```python
from build123d import *

# Parameters (mm, degrees)
SKETCH027_R     = 1.25
PAD016_DEPTH    = 5.3
SKETCH028_R     = 3.535534
SKETCH028_R_2   = 3.716517
POCKET008_DEPTH = 1.3
SKETCH032_W     = 20
SKETCH032_H     = 3
PAD019_DEPTH    = 8


with BuildPart() as part:
    # Sketch027 (on Face1 of ReferencePad002001) → Pad016 (new body)
    with BuildSketch(Plane.XY.offset(3.5)):
        Polygon((10, 124.725), (-10, 124.725), (-10, 129.975), (-25, 129.975), (-25, 134.475), (-10, 134.475), (-10, 139.725), (-10, 146.675), (10, 146.675), (10, 139.725), (10, 134.475), (25, 134.475), (25, 129.975), (10, 129.975), align=None)
        with Locations((7.5, 137.225)):
            Circle(SKETCH027_R, mode=Mode.SUBTRACT)
        with Locations((7.5, 127.225)):
            Circle(SKETCH027_R, mode=Mode.SUBTRACT)
        with Locations((-7.5, 127.225)):
            Circle(SKETCH027_R, mode=Mode.SUBTRACT)
        with Locations((-7.5, 137.225)):
            Circle(SKETCH027_R, mode=Mode.SUBTRACT)
        with Locations((-20, 132.225)):
            Circle(SKETCH027_R, mode=Mode.SUBTRACT)
        with Locations((0, 132.225)):
            Circle(SKETCH027_R, mode=Mode.SUBTRACT)
        with Locations((20, 132.225)):
            Circle(SKETCH027_R, mode=Mode.SUBTRACT)
    extrude(amount=PAD016_DEPTH)

    # Sketch028 (on Face23 of Pad016) → Pocket008 (cut)
    with BuildSketch(Plane.XY.offset(8.8)):
        with Locations((-7.5, 127.225)):
            Circle(SKETCH028_R)
        with Locations((7.5, 127.225)):
            Circle(SKETCH028_R)
        with Locations((-7.5, 137.225)):
            Circle(SKETCH028_R_2)
        with Locations((7.5, 137.225)):
            Circle(SKETCH028_R_2)
    extrude(amount=-POCKET008_DEPTH, mode=Mode.SUBTRACT)

    # Sketch032 (on Face6 of Pocket008) → Pad019 (join)
    with BuildSketch(Plane.XY.offset(8.8)):
        with Locations((0, 145.175)):
            Rectangle(SKETCH032_W, SKETCH032_H)
    extrude(amount=PAD019_DEPTH)


solid = part.part
```
Read the model definition and answer for the solid it produces. Units are mm, in the model's axes. A direction names the side the tool comes from. Give positions to 0.01 mm unless a question says otherwise; leave off trailing zeros. Write each loop counter-clockwise with the first axis right and the second up, starting at its lowest first coordinate (ties: lowest second). Pieces come first, ordered by that corner, then holes. Notation, with made-up numbers: (89.5, 15) -> (112.5, 15) arc R25 cw to (112.5, 39) -> close; hole circle Ø11 at (-1, 81). An arc over 180 degrees is marked (long way). Answer as a JSON object with one key per item and string values.
1) Section A-A on x = 0 is taken. Write down the section's boundary in (y, z) (3 decimals).
Findings below:
{"outline": "(124.725, 3.5) -> (130.975, 3.5) -> (130.975, 8.8) -> (124.725, 8.8) -> close; (133.475, 3.5) -> (146.675, 3.5) -> (146.675, 16.8) -> (143.675, 16.8) -> (143.675, 8.8) -> (133.475, 8.8) -> close"}
2) Flat-ended cylindrical pins translate along their axes: pin 1 Ø4 at (x, y) = (0, 132.225) entering from +Z; pin 2 Ø1.5 at (x, y) = (20, 132.225) entering from +Z; pin 3 Ø1 at (x, z) = (-14.5, 7.5) entering from -Y (3 decimals); pin 4 Ø3 at (x, y) = (-8, 135.5) entering from +Z. Find the tip coordinate at first contact, or state that the pin passes through.
Findings below:
{"pin 1": "stops at z = 8.8", "pin 2": "passes through", "pin 3": "stops at y = 129.975", "pin 4": "stops at z = 7.5"}
3) Section B-B on x = 7.5 is taken. Write down the section's boundary in (y, z) (3 decimals), then the cut area to 3 significant figures.
Findings below:
{"outline": "(124.725, 3.5) -> (125.975, 3.5) -> (125.975, 7.5) -> (124.725, 7.5) -> close; (128.475, 3.5) -> (135.975, 3.5) -> (135.975, 7.5) -> (133.508, 7.5) -> (133.508, 8.8) -> (130.761, 8.8) -> (130.761, 7.5) -> (128.475, 7.5) -> close; (138.475, 3.5) -> (146.675, 3.5) -> (146.675, 16.8) -> (143.675, 16.8) -> (143.675, 8.8) -> (140.942, 8.8) -> (140.942, 7.5) -> (138.475, 7.5) -> close", "area": "103 mm^2"}
4) Section C-C on z = 6.75 is taken. Write down the section's boundary in (x, y) (3 decimals).
Findings below:
{"outline": "(-25, 129.975) -> (-10, 129.975) -> (-10, 124.725) -> (10, 124.725) -> (10, 129.975) -> (25, 129.975) -> (25, 134.475) -> (10, 134.475) -> (10, 146.675) -> (-10, 146.675) -> (-10, 134.475) -> (-25, 134.475) -> close; hole circle Ø2.5 at (-20, 132.225); hole circle Ø2.5 at (-7.5, 127.225); hole circle Ø2.5 at (-7.5, 137.225); hole circle Ø2.5 at (0, 132.225); hole circle Ø2.5 at (7.5, 127.225); hole circle Ø2.5 at (7.5, 137.225); hole circle Ø2.5 at (20, 132.225)"}
5) Section D-D on x = -20 is taken. Write down the section's boundary in (y, z) (3 decimals).
Findings below:
{"outline": "(129.975, 3.5) -> (130.975, 3.5) -> (130.975, 8.8) -> (129.975, 8.8) -> close; (133.475, 3.5) -> (134.475, 3.5) -> (134.475, 8.8) -> (133.475, 8.8) -> close"}
6) For a pull along Y with two mould halves and no side action, classify faces 4 (the flat face through (-17, 129.975, 6)), 5 (the cylindrical face through (19.837, 133.464, 6.113)), 6 (the flat face through (0, 134, 8.8)) as pulls with the +Y half, pulls with the -Y half, needs draft (parallel to the pull), parting line crosses it, or undercut.
Findings below:
{"face 4": "pulls with the -Y half", "face 5": "undercut", "face 6": "needs draft"}
7) A tool of negligible diameter and unlimited length cuts with its end or side. For faces 1 (the flat face through (-18, 134.475, 6)), 2 (the flat face through (6, 128, 7.5)), 3 (the flat face through (0, 143.675, 13)), from which of +Z, -Z, +X, -X, +Y, -Y can it reach the whole face along a straight path? Write none if from no direction.
Findings below:
{"face 1": "+Z, -Z, -X, +Y", "face 2": "+Z", "face 3": "+Z, +X, -X, -Y"}
8) Straight lines are drawn through the part: probe 1 along Y at (x, z) = (7.5, 4.7) (3 decimals); probe 2 along Y at (x, z) = (20, 6.2) (3 decimals); probe 3 along X at (y, z) = (131.25, 5.25). For each, find the intervals that lie inside material, in ascending order. Write a range as from..to.
Findings below:
{"probe 1": "y = 124.725..125.975, 128.475..135.975, 138.475..146.675", "probe 2": "y = 129.975..130.975, 133.475..134.475", "probe 3": "x = -25..-20.78, -19.22..-0.78, 0.78..19.22, 20.78..25"}
